Answer from the drawing. Dimensions are ordinates in mm from the lowest x, y and z of the part. A direction names the side the tool comes from. Coordinates: 2 decimals unless noted, no trailing zeros. Loops run counter-clockwise (first coordinate to the right, second up) from the corner with the lowest first, then second, coordinate; pieces in that order, holes last. Notation, with made-up numbers: (72, 50) -> (101, 50) arc R16 ccw to (101, 65) -> close; hole circle Ø9 at (-32.5, -7.75). An arc over 180 degrees is marked (long way). Use a Markdown table: item, result.
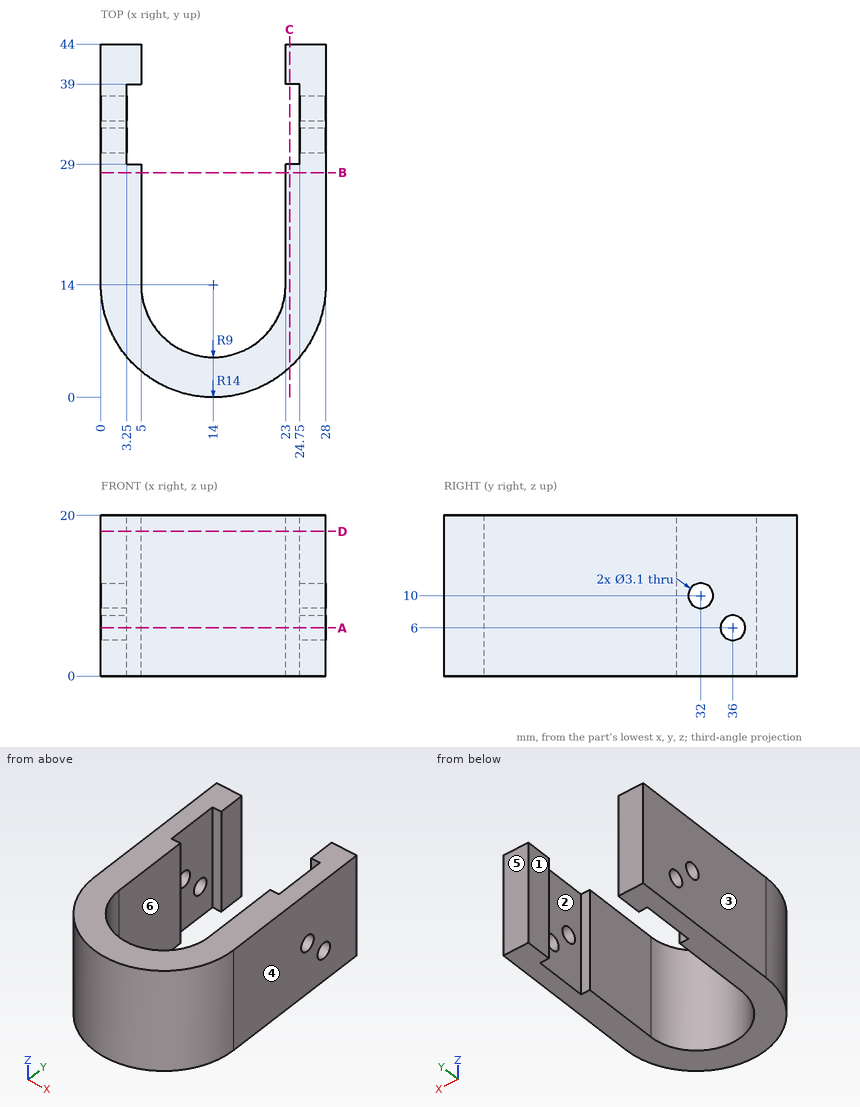
Q1. Section B-B on y = 28 is taken. Determine the outline of the cut face in (x, z), and give its area (3 significant figures).
Solved:
| item | result |
|---|---|
| outline | (0, 0) -> (5, 0) -> (5, 20) -> (0, 20) -> close; (23, 0) -> (28, 0) -> (28, 20) -> (23, 20) -> close |
| area | 200 mm² |
Q2. Section A-A on z = 6 is taken. Determine the outline of the cut face in (x, y).
Solved:
| item | result |
|---|---|
| outline | (0, 14) arc R14 ccw to (28, 14) -> (28, 34.45) -> (24.75, 34.45) -> (24.75, 29) -> (23, 29) -> (23, 14) arc R9 cw to (5, 14) -> (5, 29) -> (3.25, 29) -> (3.25, 34.45) -> (0, 34.45) -> close; (0, 37.55) -> (3.25, 37.55) -> (3.25, 39) -> (5, 39) -> (5, 44) -> (0, 44) -> close; (23, 39) -> (24.75, 39) -> (24.75, 37.55) -> (28, 37.55) -> (28, 44) -> (23, 44) -> close |
Q3. Section C-C on x = 23.5 is taken. Determine the outline of the cut face in (y, z).
Solved:
| item | result |
|---|---|
| outline | (3.72, 0) -> (29, 0) -> (29, 20) -> (3.72, 20) -> close; (39, 0) -> (44, 0) -> (44, 20) -> (39, 20) -> close |
Q4. For the marked faces 1, 2 and 3, determine the directions among +Z, -Z, +X, -X, +Y, -Y from which every point of the face is accessible in a straight line to the end or side of a thin tool.
Solved:
| item | result |
|---|---|
| face 1 | +Z, -Z, +Y |
| face 2 | +Z, -Z |
| face 3 | +Z, -Z, -X, +Y, -Y |
Q5. Given pin 1 Ø1 at (x, z) = (24, 4.5) entering from -Y; pin 2 Ø1.4 at (x, z) = (4.5, 15) entering from -Y; pin 3 Ø6 at (x, z) = (9, 10.5) entering from -Y; pin 4 Ø12 at (x, y) = (13.5, 25.5) entering from -Z, each flat-ended and moving along its own axis, determine where each tip first touches the part or whether it passes through.
Solved:
| item | result |
|---|---|
| pin 1 | y = 3.72 |
| pin 2 | y = 3.11 |
| pin 3 | y = 0.14 |
| pin 4 | through |
Q6. Section D-D on z = 18 is taken. Determine the outline of the cut face in (x, y).
Solved:
| item | result |
|---|---|
| outline | (0, 14) arc R14 ccw to (28, 14) -> (28, 44) -> (23, 44) -> (23, 39) -> (24.75, 39) -> (24.75, 29) -> (23, 29) -> (23, 14) arc R9 cw to (5, 14) -> (5, 29) -> (3.25, 29) -> (3.25, 39) -> (5, 39) -> (5, 44) -> (0, 44) -> close |
Q7. Determine the mould class of the marked faces 4, 5 and 6 for opening direction X: pulls with the +X half, pulls with the -X half, needs draft (parallel to the pull), parting line crosses it, or undercut.
Solved:
| item | result |
|---|---|
| face 4 | pulls with the +X half |
| face 5 | needs draft |
| face 6 | undercut |
Q8. Consider line 1 (X direction, y = 16, z = 16.75); line 2 (X direction, y = 29.5, z = 13); line 3 (Z direction, x = 2.5, y = 35). Determine where each line is inside the solid, lowest interval first. Write a range as [from, to].
Solved:
| item | result |
|---|---|
| line 1 | [0, 5], [23, 28] |
| line 2 | [0, 3.25], [24.75, 28] |
| line 3 | [0, 4.82], [7.18, 20] |
